```python
from build123d import *

# Parameters (mm, degrees)
SKETCH_1_R          = 3.515
EXTRUDE_1_DEPTH     = 4
FILLET_1_R          = 10
CHAMFER_1_SIZE      = 0.2
SKETCH_3_R          = 4.15
CUT_EXTRUDE_2_DEPTH = 0.1
SKETCH_4_R          = 4.125
CUT_EXTRUDE_3_DEPTH = 0.1


with BuildPart() as part:
    # 草图1 → 凸台-拉伸1 (new body)
    with BuildSketch(Plane(origin=(0, 0, 0), x_dir=(1, 0, 0), z_dir=(0, 1, 0))):
        with BuildLine():
            Line((4.898979486, 2.5), (115.101020514, 2.5))
            ThreePointArc((115.101020514, 2.5), (125.5, 0), (115.101020514, -2.5))
            Line((115.101020514, -2.5), (4.898979486, -2.5))
            ThreePointArc((4.898979486, -2.5), (-5.5, 0), (4.898979486, 2.5))
        make_face()
        with Locations(Location((0, 0, 0), (0, 0, 270))):
            Circle(SKETCH_1_R, mode=Mode.SUBTRACT)
        with Locations(Location((120, 0, 0), (0, 0, 270))):
            Circle(SKETCH_1_R, mode=Mode.SUBTRACT)
    extrude(amount=EXTRUDE_1_DEPTH)

    # 圆角1
    fillet_1_edges = [part.edges().sort_by_distance(p)[0] for p in [
        (4.898979486, 2, -2.5),
        (115.101020514, 2, -2.5),
        (115.101020514, 2, 2.5),
        (4.898979486, 2, 2.5),
    ]]
    fillet(fillet_1_edges, radius=FILLET_1_R)

    # 倒角1
    chamfer_1_edges = [part.edges().sort_by_distance(p)[0] for p in [
        (125.5, 0, 0),
        (125.5, 4, 0),
        (60, 0, 2.5),
        (60, 4, 2.5),
        (60, 0, -2.5),
        (60, 4, -2.5),
        (-5.5, 0, 0),
        (-5.5, 4, 0),
        (113.945703694, 0, 2.996180734),
        (113.945703694, 4, 2.996180734),
        (113.945703694, 0, -2.996180734),
        (113.945703694, 4, -2.996180734),
        (6.054296306, 0, 2.996180734),
        (6.054296306, 4, 2.996180734),
        (6.054296306, 0, -2.996180734),
        (6.054296306, 4, -2.996180734),
    ]]
    chamfer(chamfer_1_edges, length=CHAMFER_1_SIZE)

    # 草图3 → 切除-拉伸2 (cut)
    with BuildSketch(Plane(origin=(0, 4, 0), x_dir=(1, 0, 0), z_dir=(0, 1, 0))):
        with Locations(Location((0, 0, 0), (0, 0, 270))):
            Circle(SKETCH_3_R)
        with Locations(Location((120, 0, 0), (0, 0, 270))):
            Circle(SKETCH_3_R)
    extrude(amount=-CUT_EXTRUDE_2_DEPTH, mode=Mode.SUBTRACT)

    # 草图4 → 切除-拉伸3 (cut)
    with BuildSketch(Plane.XZ):
        with Locations(Location((0, 0, 0), (0, 0, 270))):
            Circle(SKETCH_4_R)
        with Locations(Location((120, 0, 0), (0, 0, 270))):
            Circle(SKETCH_4_R)
    extrude(amount=-CUT_EXTRUDE_3_DEPTH, mode=Mode.SUBTRACT)


solid = part.part
```
The model under review builds one solid part; all positions refer to its coordinate system, in mm. A direction names the side the tool comes from. Coordinates: 2 decimals unless noted, no trailing zeros. Write each loop counter-clockwise with the first axis right and the second up, starting at its lowest first coordinate (ties: lowest second). Pieces come first, ordered by that corner, then holes.
1) We need section C-C on y = 2.85. State the section outline as (x, z) points (3 decimals).
2) We need section D-D on x = 78. State the section outline as (y, z) points.
3) We need section A-A on x = 120. State the section outline as (y, z) points (3 decimals).
4) We need section B-B on z = 0. Count the separate pieces of the cut face and the enclosed holes in it, then the cut area to 3 significant figures.
5) The part is to be moulded in two halves that separate along Z. For faces 4 (the face through (61, 0, 0)), 5 (the face through (113.9, 2.03, -2.98)), 6 (the face through (113.99, 2.03, 3.01)), 7 (the face through (116.57, 1.97, -0.76)), say which applies: pulls with the +Z half, pulls with the -Z half, needs draft (parallel to the pull), parting line crosses it, or undercut.
6) Clearance check with flat-ended pins moving along their axes: pin 1 Ø2 at (x, y) = (32.5, 3) entering from +Z; pin 2 Ø2 at (y, z) = (1.5, 4) entering from -X. State where each tip first meets the part, or that it passes through.
7) Machinability: for faces 1 (the face through (59, 2, -2.5)), 2 (the face through (-5.497, 1.975, 0.17)), 3 (the face through (6.01, 2.03, 3.01)), which of the approach directions +Z, -Z, +X, -X, +Y, -Y give a long, thin tool a straight path to every point of the face, cutting with its end or side? Answer none if there is none.
8) To check wall thickness, follow probe 1 along X at (y, z) = (1.7, -0.75); probe 2 along Z at (x, y) = (120, 2.25) (3 decimals); probe 3 along X at (y, z) = (2.9, 0) (3 decimals). State the ranges of each line that lie inside material, in increasing order.
Answer list:
1. outline: (3.252, -4.435) arc R10 cw to (9.165, -2.5) - (110.835, -2.5) arc R10 cw to (116.748, -4.435) arc R5.5 ccw (long way) to (116.748, 4.435) arc R10 cw to (110.835, 2.5) - (9.165, 2.5) arc R10 cw to (3.252, 4.435) arc R5.5 ccw (long way) to start; hole circle Ø7.03 at (0, 0); hole circle Ø7.03 at (120, 0)
2. outline: (0, -2.3) - (0.2, -2.5) - (3.8, -2.5) - (4, -2.3) - (4, 2.3) - (3.8, 2.5) - (0.2, 2.5) - (0, 2.3) - close
3. outline: (0, -5.3) - (0.2, -5.5) - (3.8, -5.5) - (4, -5.3) - (4, -4.15) - (3.9, -4.15) - (3.9, -3.515) - (0.1, -3.515) - (0.1, -4.125) - (0, -4.125) - close; (0, 4.125) - (0.1, 4.125) - (0.1, 3.515) - (3.9, 3.515) - (3.9, 4.15) - (4, 4.15) - (4, 5.3) - (3.8, 5.5) - (0.2, 5.5) - (0, 5.3) - close
4. separate pieces: 3
4. enclosed holes: 0
4. area: 467 mm2
5. face 4: needs draft
5. face 5: pulls with the -Z half
5. face 6: pulls with the +Z half
5. face 7: undercut
6. pin 1: stops at z = 2.5
6. pin 2: stops at x = -4.61
7. face 1: -Z, +Y, -Y
7. face 2: +Y, -Y
7. face 3: +Z, +Y, -Y
8. probe 1: x = -5.45 to -3.43, 3.43 to 116.57, 123.43 to 125.45
8. probe 2: z = -5.5 to -3.515, 3.515 to 5.5
8. probe 3: x = -5.5 to -3.515, 3.515 to 116.485, 123.515 to 125.5
